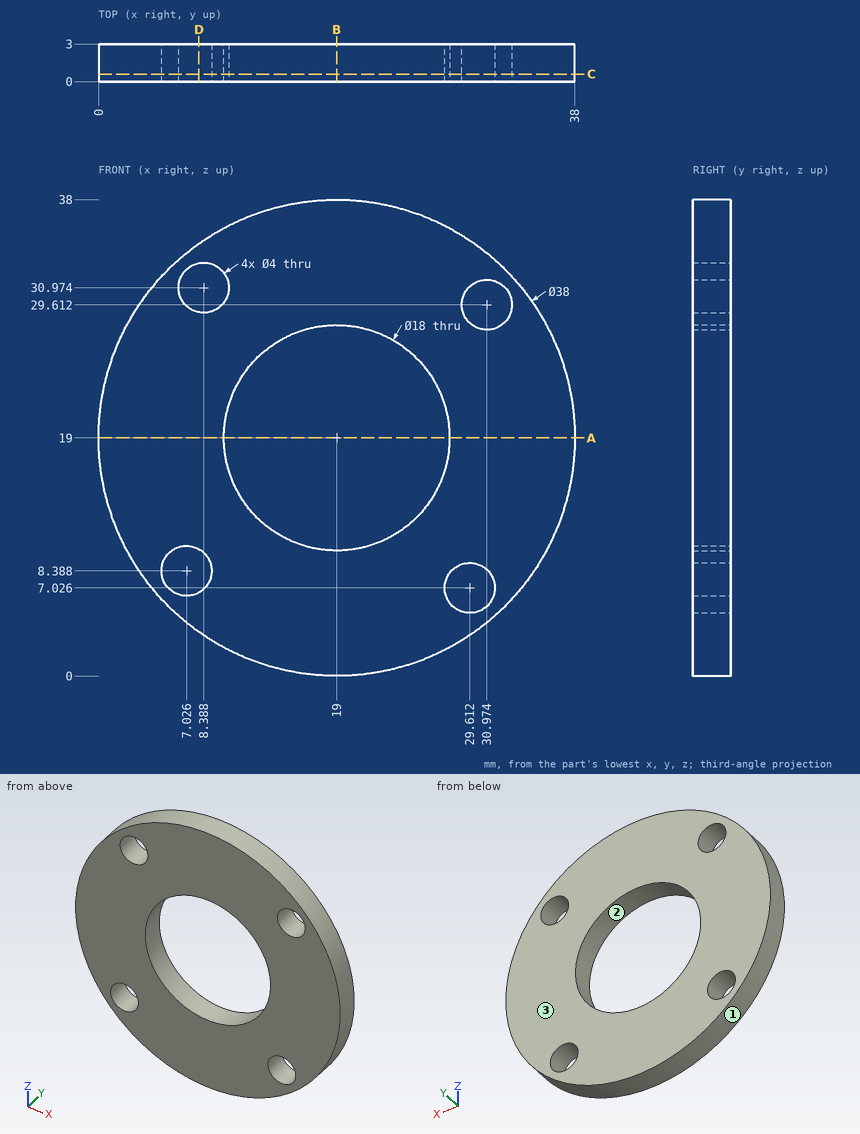
Can you work these out from the drawing? Everything is in mm from the part's minimum corner. Round coordinates to 2 decimals unless told otherwise and drop trailing zeros. Loops run counter-clockwise (first coordinate to the right, second up) from the corner with the lowest first, then second, coordinate; pieces in that order, holes last. Notation, with made-up numbers: (65, 18.25) -> (91, 18.25) arc R29 ccw to (91, 50.25) -> close; hole circle Ø11 at (31.25, -29.5). An arc over 180 degrees is marked (long way). Use CSV: the item, a comma, the result in double quotes.
(1) Suppose I cut it at B-B on x = 19. Write out the boundary of the cut face in (y, z).
Return value:
outline,"(0, 0) -> (3, 0) -> (3, 10) -> (0, 10) -> close; (0, 28) -> (3, 28) -> (3, 38) -> (0, 38) -> close"
(2) Suppose I cut it at C-C on y = 0.6. Write out the boundary of the cut face in (x, z) (1 decimal).
Return value:
outline,"circle Ø38 at (19, 19); hole circle Ø4 at (7, 8.4); hole circle Ø4 at (8.4, 31); hole circle Ø18 at (19, 19); hole circle Ø4 at (29.6, 7); hole circle Ø4 at (31, 29.6)"
(3) If we mould it in two halves opening along X, with no side actions, what happens to the marked faces 1, 2 and 3? For each: +X half, -X half, draft (parallel to the pull), parting line (faces both ways), or undercut.
Return value:
face 1,"parting line"
face 2,"undercut"
face 3,"draft"
(4) If I drill on probe 1 along Z at (x, y) = (19, 2.15); probe 2 along Z at (x, y) = (8.5, 2) (1 decimal); probe 3 along Z at (x, y) = (29.5, 2.15) (1 decimal), over which ranges is the centre line in solid material (lowest first)? Write a range as [from, to].
Return value:
probe 1,"z = [0, 10], [28, 38]"
probe 2,"z = [3.2, 7], [9.7, 29], [33, 34.8]"
probe 3,"z = [3.2, 5], [9, 28.3], [31, 34.8]"
(5) Will these pins go through, and if not, where does the flat tip stop? pin 1 Ø1 at (x, y) = (23.5, 0.5) entering from +Z (1 decimal); pin 2 Ø5 at (x, z) = (5, 21) entering from -Y; pin 3 Ø1 at (y, z) = (2, 22) entering from +X (1 decimal); pin 4 Ø1.5 at (x, y) = (8.5, 2) entering from +Z.
Return value:
pin 1,"stops at z = 37.6"
pin 2,"stops at y = 0"
pin 3,"stops at x = 37.8"
pin 4,"stops at z = 35.31"
(6) Suppose I cut it at D-D on x = 8. Write out the boundary of the cut face in (y, z) (1 decimal).
Return value:
outline,"(0, 3.5) -> (3, 3.5) -> (3, 6.6) -> (0, 6.6) -> close; (0, 10.1) -> (3, 10.1) -> (3, 29) -> (0, 29) -> close; (0, 32.9) -> (3, 32.9) -> (3, 34.5) -> (0, 34.5) -> close"
(7) Suppose I cut it at A-A on z = 19. Write out the boundary of the cut face in (x, y).
Return value:
outline,"(0, 0) -> (10, 0) -> (10, 3) -> (0, 3) -> close; (28, 0) -> (38, 0) -> (38, 3) -> (28, 3) -> close"
